Here's the drawing with two shaded views (mm, measured from the low corner). I have some questions. Round coordinates to 2 decimals unless told otherwise and drop trailing zeros. Loops run counter-clockwise (first coordinate to the right, second up) from the corner with the lowest first, then second, coordinate; pieces in that order, holes last. Notation, with made-up numbers: M 29,61 L 53,61 A16 ccw 53,86 Z; hole C 53.5,-28.75 d3. An arc over 180 degrees is marked long. One line per item, written item: value. Start each with the question number.
Q1. Imagine slicing it at C-C (x = 68.5). Please give me the cut outline in (y, z), then the cut area to 3 significant figures.
Q2. Imagine slicing it at D-D (z = 3.75). Please give me the cut outline in (x, y).
Q3. Imagine slicing it at A-A (x = 43.5). Please give me the cut outline in (y, z).
Q4. Please list where these lines run through material, in increasing order: line 1 along Y through (x, z) = (43.5, 3.5); line 2 along X through (y, z) = (73, 4.25); line 3 along X through (y, z) = (12, 4).
Q5. I'm going to push a flat-ended pin straight in: pin 1 Ø3.5 at (x, y) = (18.5, 75) entering from -Z. Where does the tip first touch, or does it pass through?
Q6. Imagine slicing it at B-B (y = 65.4). Please give me the cut outline in (x, z), then the cut area to 3 significant figures.
Q7. Thinking about a two-plate mould opening in Z: for the marked faces 1 and 2, which applies, released by +Z, released by -Z, zero draft, split by the parting line, or undercut?
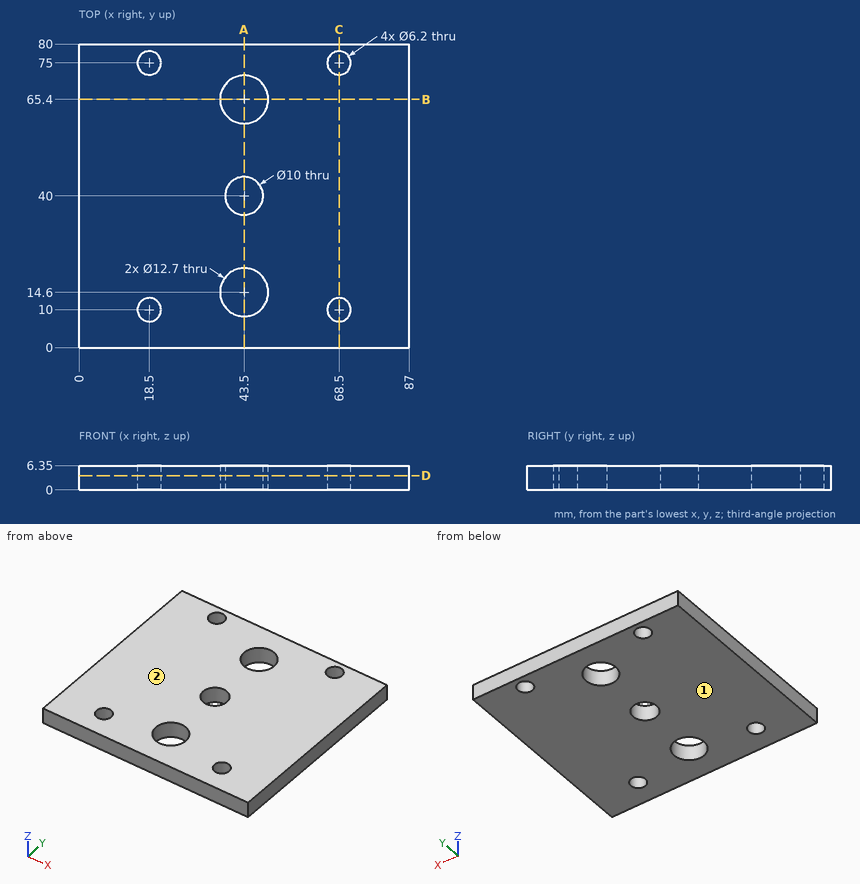
Report:
1. outline: M 0,0 L 6.9,0 L 6.9,6.35 L 0,6.35 Z; M 13.1,0 L 71.9,0 L 71.9,6.35 L 13.1,6.35 Z; M 78.1,0 L 80,0 L 80,6.35 L 78.1,6.35 Z
1. area: 429 mm²
2. outline: M 0,0 L 87,0 L 87,80 L 0,80 Z; hole C 18.5,10 d6.2; hole C 18.5,75 d6.2; hole C 43.5,14.6 d12.7; hole C 43.5,65.4 d12.7; hole C 43.5,40 d10; hole C 68.5,10 d6.2; hole C 68.5,75 d6.2
3. outline: M 0,0 L 8.25,0 L 8.25,6.35 L 0,6.35 Z; M 20.95,0 L 35,0 L 35,6.35 L 20.95,6.35 Z; M 45,0 L 59.05,0 L 59.05,6.35 L 45,6.35 Z; M 71.75,0 L 80,0 L 80,6.35 L 71.75,6.35 Z
4. line 1: y = 0 to 8.25, 20.95 to 35, 45 to 59.05, 71.75 to 80
4. line 2: x = 0 to 16.13, 20.87 to 66.13, 70.87 to 87
4. line 3: x = 0 to 16.13, 20.87 to 37.71, 49.29 to 66.13, 70.87 to 87
5. pin 1: passes through
6. outline: M 0,0 L 37.15,0 L 37.15,6.35 L 0,6.35 Z; M 49.85,0 L 87,0 L 87,6.35 L 49.85,6.35 Z
6. area: 472 mm²
7. face 1: released by -Z
7. face 2: released by +Z
